from build123d import *

# Parameters (mm, degrees)
BOSS_EXTRUDE1_DEPTH = 3
SKETCH2_R           = 3
SKETCH2_R_2         = 1.5
BOSS_EXTRUDE2_DEPTH = 10
SKETCH3_R           = 2
SKETCH3_R_2         = 1.5
CUT_EXTRUDE1_DEPTH  = 101.928192295
SKETCH4_W           = 6
SKETCH4_H           = 10
BOSS_EXTRUDE3_DEPTH = 18.5
SKETCH5_W           = 6
SKETCH5_H           = 10
CUT_EXTRUDE2_DEPTH  = 159.159729388
CHAMFER1_SIZE       = 6
FILLET1_START       = -61
FILLET1_DEPTH       = 6
FILLET1_START_2     = 55
FILLET1_2_DEPTH     = 6


with BuildPart() as part:
    # Sketch1 → Boss-Extrude1 (new body)
    with BuildSketch(Plane(origin=(0, 0, 0), x_dir=(1, 0, 0), z_dir=(0, 1, 0))):
        Polygon((30, -50), (30, -40), (30, 40), (30, 50), (-30, 50), (-30, 40), (-30, -40), (-30, -50), align=None)
        Polygon((-87.5, -31), (-30, -40), (-30, 40), (-87.5, 31), align=None)
        Polygon((30, 40), (30, -40), (87.5, -31), (87.5, 31), align=None)
    extrude(amount=BOSS_EXTRUDE1_DEPTH)

    # Sketch2 → Boss-Extrude2 (add)
    # profile 1 of 2: a face of its own
    with BuildSketch(Plane.XY.offset(50)):
        with Locations((19, 5.5)):
            Circle(SKETCH2_R)
        with Locations((19, 5.5)):
            Circle(SKETCH2_R_2, mode=Mode.SUBTRACT)
    # profile 2 of 2: a face of its own
    with BuildSketch(Plane.XY.offset(50)):
        with Locations((-19, 5.5)):
            Circle(SKETCH2_R)
        with Locations(Location((-19, 5.5, 0), (0, 0, 180))):
            Circle(SKETCH2_R_2, mode=Mode.SUBTRACT)
    boss_extrude2 = extrude(amount=-BOSS_EXTRUDE2_DEPTH)

    # Mirror1: Boss-Extrude2 across plane
    add(boss_extrude2.mirror(Plane.XY))

    # Sketch3 → Cut-Extrude1 (cut, through all)
    with BuildSketch(Plane(origin=(0, 3, 0), x_dir=(1, 0, 0), z_dir=(0, 1, 0))):
        with Locations(Location((0, 0, 0), (0, 0, 270))):
            Circle(SKETCH3_R)
        with Locations(Location((10, 27, 0), (0, 0, 270))):
            Circle(SKETCH3_R_2)
        with Locations(Location((-10, 27, 0), (0, 0, 90))):
            Circle(SKETCH3_R_2)
        with Locations(Location((10, -27, 0), (0, 0, 90))):
            Circle(SKETCH3_R_2)
        with Locations(Location((-10, -27, 0), (0, 0, 270))):
            Circle(SKETCH3_R_2)
        with BuildLine():
            Line((30.5, 26), (40.5, 26))
            ThreePointArc((40.5, 26), (42, 24.5), (40.5, 23))
            Line((40.5, 23), (30.5, 23))
            ThreePointArc((30.5, 23), (29, 24.5), (30.5, 26))
        make_face()
        with BuildLine():
            Line((-30.5, 26), (-40.5, 26))
            ThreePointArc((-40.5, 26), (-42, 24.5), (-40.5, 23))
            Line((-40.5, 23), (-30.5, 23))
            ThreePointArc((-30.5, 23), (-29, 24.5), (-30.5, 26))
        make_face()
        with BuildLine():
            Line((30.5, -26), (40.5, -26))
            ThreePointArc((40.5, -26), (42, -24.5), (40.5, -23))
            Line((40.5, -23), (30.5, -23))
            ThreePointArc((30.5, -23), (29, -24.5), (30.5, -26))
        make_face()
        with BuildLine():
            Line((-30.5, -26), (-40.5, -26))
            ThreePointArc((-40.5, -26), (-42, -24.5), (-40.5, -23))
            Line((-40.5, -23), (-30.5, -23))
            ThreePointArc((-30.5, -23), (-29, -24.5), (-30.5, -26))
        make_face()
    extrude(amount=-CUT_EXTRUDE1_DEPTH, mode=Mode.SUBTRACT)

    # Sketch4 → Boss-Extrude3 (add)
    with BuildSketch(Plane(origin=(0, 3, 0), x_dir=(1, 0, 0), z_dir=(0, 1, 0))):
        with Locations((58, 22.5)):
            Rectangle(SKETCH4_W, SKETCH4_H)
        with Locations((58, -22.5)):
            Rectangle(SKETCH4_W, SKETCH4_H)
        with Locations((-58, -22.5)):
            Rectangle(SKETCH4_W, SKETCH4_H)
        with Locations((-58, 22.5)):
            Rectangle(SKETCH4_W, SKETCH4_H)
    extrude(amount=BOSS_EXTRUDE3_DEPTH)

    # Sketch5 → Cut-Extrude2 (cut, through all)
    with BuildSketch(Plane.ZY.offset(61)):
        with Locations((-20.5, 16.5)):
            Rectangle(SKETCH5_W, SKETCH5_H)
        with Locations((20.5, 16.5)):
            Rectangle(SKETCH5_W, SKETCH5_H)
    extrude(amount=-CUT_EXTRUDE2_DEPTH, mode=Mode.SUBTRACT)

    # Chamfer1
    chamfer1_edges = [part.edges().sort_by_distance(p)[0] for p in [
        (58, 11.5, 17.5),
        (-58, 11.5, 17.5),
        (58, 11.5, -17.5),
        (-58, 11.5, -17.5),
    ]]
    chamfer(chamfer1_edges, length=CHAMFER1_SIZE - 0.0001)  # a hair under: the kernel refuses the full size

    # Fillet1: read off the stored shape, not the designer's step
    # Fillet1 outline → Fillet1 (add)
    with BuildSketch(Plane.YZ.offset(FILLET1_START)):
        with BuildLine():
            ThreePointArc((13.571067812, -23.5), (11.65765065, -23.119397663), (10.035533906, -22.035533906))
            Line((10.035533906, -22.035533906), (11.5, -23.5))
            Line((11.5, -23.5), (13.571067812, -23.5))
        make_face()
        with BuildLine():
            ThreePointArc((10.035533906, 22.035533906), (11.65765065, 23.119397663), (13.571067812, 23.5))
            Line((13.571067812, 23.5), (11.5, 23.5))
            Line((11.5, 23.5), (10.035533906, 22.035533906))
        make_face()
    extrude(amount=FILLET1_DEPTH)

    # Fillet1 2 outline → Fillet1 2 (add)
    with BuildSketch(Plane.YZ.offset(FILLET1_START_2)):
        with BuildLine():
            ThreePointArc((13.571067812, -23.5), (11.65765065, -23.119397663), (10.035533906, -22.035533906))
            Line((10.035533906, -22.035533906), (11.5, -23.5))
            Line((11.5, -23.5), (13.571067812, -23.5))
        make_face()
        with BuildLine():
            ThreePointArc((10.035533906, 22.035533906), (11.65765065, 23.119397663), (13.571067812, 23.5))
            Line((13.571067812, 23.5), (11.5, 23.5))
            Line((11.5, 23.5), (10.035533906, 22.035533906))
        make_face()
    extrude(amount=FILLET1_2_DEPTH)


solid = part.part
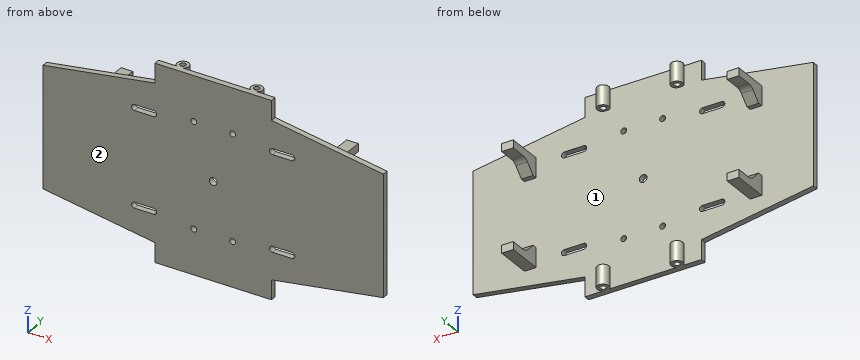
The model under review builds one solid part; all positions refer to its coordinate system, in mm. Face numbers are marked on the shaded views. Coordinates: 2 decimals unless noted, no trailing zeros. Loops run counter-clockwise (first coordinate to the right, second up) from the corner with the lowest first, then second, coordinate; pieces in that order, holes last.
(1) Draft analysis for pull direction Z (two halves, no side actions). For the marked faces 1 and 2, state which applies: +Z half, -Z half, draft (parallel to the pull), parting line (faces both ways), or undercut.
Determined:
face 1: undercut
face 2: draft
(2) Insertion check: P1, Ø3, axis at y = 9.5, z = 21.5, coming from the -X side; P2, Ø0.8, axis at x = 57, y = 4, coming from the +Z side; P3, Ø5, axis at y = 11, z = 23.5, coming from the +X side; P4, Ø3, axis at x = 0, z = 0, coming from the +Y side. Each pin has a flat end and moves straight along its axis. Give the tip position at first contact, or say it passes through.
Determined:
P1: stops at x = -61
P2: stops at z = 27.5
P3: stops at x = 61
P4: passes through
(3) Consider section B-B, the plane z = 13.5. Give the boundary of the cut face in (x, y).
Determined:
outline: (-87.5, 0) - (87.5, 0) - (87.5, 3) - (-87.5, 3) - close
(4) Consider section C-C, the plane x = -49. Give the boundary of the cut face in (y, z), plus the area to 3 significant figures.
Determined:
outline: (0, -37.03) - (3, -37.03) - (3, 37.03) - (0, 37.03) - close
area: 222 mm2
(5) Consider section A-A, the plane y = 18.5. Give the boundary of the cut face in (x, z), plus the area to 3 significant figures.
Determined:
outline: (-61, -27.5) - (-55, -27.5) - (-55, -23.5) - (-61, -23.5) - close; (-61, 23.5) - (-55, 23.5) - (-55, 27.5) - (-61, 27.5) - close; (55, -27.5) - (61, -27.5) - (61, -23.5) - (55, -23.5) - close; (55, 23.5) - (61, 23.5) - (61, 27.5) - (55, 27.5) - close
area: 96.0 mm2
(6) Wall thickness on L1, parallel to X at y = 1.85, z = 27; L2, parallel to Y at x = 19, z = -44.25; L3, parallel to Y at x = 3, z = -18: over which ranges is each line inside the solid? List them lowest first.
Determined:
L1: x = -87.5 to -11.5, -8.5 to 8.5, 11.5 to 87.5
L2: y = 0 to 4, 7 to 8.5
L3: y = 0 to 3
